```python
from build123d import *

# Parameters (mm, degrees)
BOSS_EXTRUDE1_DEPTH = 7.9375
SKETCH2_R           = 5.207
CUT_EXTRUDE1_DEPTH  = 3.96875


with BuildPart() as part:
    # Sketch1 → Boss-Extrude1 (new, symmetric)
    with BuildSketch(Plane(origin=(0, 0, 0), x_dir=(1, 0, 0), z_dir=(0, 1, 0))):
        Polygon((0, 0), (3.96875, 0), (120.93575, 0), (120.93575, 3.96875), (3.96875, 3.96875), (3.96875, 75.34275), (0, 75.34275), align=None)
    extrude(amount=BOSS_EXTRUDE1_DEPTH, both=True)

    # Sketch2 → Cut-Extrude1 (cut)
    with BuildSketch(Plane.XY):
        with Locations((47.4345, 0)):
            Circle(SKETCH2_R)
    extrude(amount=-CUT_EXTRUDE1_DEPTH, mode=Mode.SUBTRACT)


solid = part.part
```
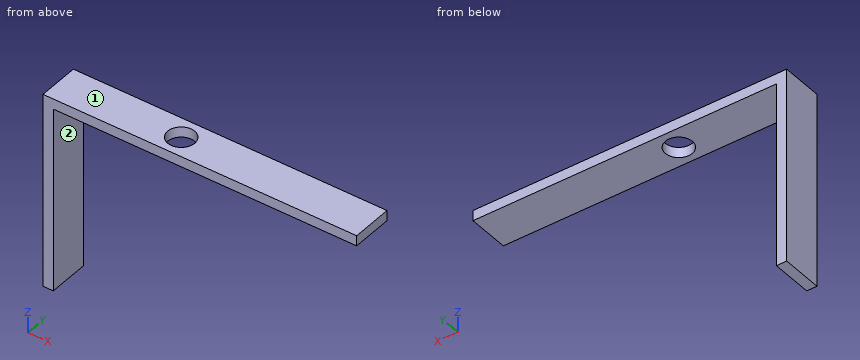
Can you work these out from the model? Positions are in its coordinate system, mm. Face numbers are marked on the shaded views. A direction names the side the tool comes from. Coordinates: 2 decimals unless noted, no trailing zeros. Loops run counter-clockwise (first coordinate to the right, second up) from the corner with the lowest first, then second, coordinate; pieces in that order, holes last. Notation, with made-up numbers: (12.25, 84) - (21.25, 84) arc R12 ccw to (21.25, 99) - close; hole circle Ø9 at (18.25, -26). An arc over 180 degrees is marked (long way). Use a Markdown table: item, result.
Item 1: I want a section at A-A on y = 0. Please give me the cut outline in (x, z).
Numbers:
| item | result |
|---|---|
| outline | (0, -75.34) - (3.97, -75.34) - (3.97, -3.97) - (42.23, -3.97) - (42.23, 0) - (0, 0) - close; (52.64, -3.97) - (120.94, -3.97) - (120.94, 0) - (52.64, 0) - close |
Item 2: I want a section at D-D on x = 15.5. Please give me the cut outline in (y, z).
Numbers:
| item | result |
|---|---|
| outline | (-7.94, -3.97) - (7.94, -3.97) - (7.94, 0) - (-7.94, 0) - close |
Item 3: I want a section at B-B on x = 46. Please give me the cut outline in (y, z), and give its area (3 significant figures).
Numbers:
| item | result |
|---|---|
| outline | (-7.94, -3.97) - (-5.01, -3.97) - (-5.01, 0) - (-7.94, 0) - close; (5.01, -3.97) - (7.94, -3.97) - (7.94, 0) - (5.01, 0) - close |
| area | 23.3 mm2 |
Item 4: For the marked faces 1 and 2, which set-ups out of +Z, -Z, +X, -X, +Y, -Y let a thin tool reach every point of the face, with its end or its side?
Numbers:
| item | result |
|---|---|
| face 1 | +Z, +X, -X, +Y, -Y |
| face 2 | -Z, +X, +Y, -Y |
Item 5: I want a section at C-C on z = -42.5. Please give me the cut outline in (x, y), and give its area (3 significant figures).
Numbers:
| item | result |
|---|---|
| outline | (0, -7.94) - (3.97, -7.94) - (3.97, 7.94) - (0, 7.94) - close |
| area | 63.0 mm2 |
Item 6: Will this pin go through, and if not, where does the flat tip stop? pin 1 (8 mm diameter, centred on x = 54.5, y = -2.5, fed in from -Z).
Numbers:
| item | result |
|---|---|
| pin 1 | stops at z = -3.97 |
Item 7: If I drill on probe 1 along X at (y, z) = (6.25, -71); probe 2 along Z at (x, y) = (76.5, 5), over which ranges is the centre line in solid material (lowest first)? Write a range as from..to.
Numbers:
| item | result |
|---|---|
| probe 1 | x = 0..3.97 |
| probe 2 | z = -3.97..0 |
